Read the model definition and answer for the solid it produces. Units are mm, in the model's axes. Coordinates: 2 decimals unless noted, no trailing zeros. Write each loop counter-clockwise with the first axis right and the second up, starting at its lowest first coordinate (ties: lowest second). Pieces come first, ordered by that corner, then holes.
Item 1: Determine the mould class of faces 1 (the face through (1.02, 46.49, 1.97)), 2 (the face through (29.23, -26.81, 1.97)), 3 (the face through (-11, -10, 0)) for opening direction Y: released by +Y, released by -Y, zero draft, split by the parting line, or undercut.
Item 2: Each of these flat-tipped pins is pushed along its axis until it touches: P1, Ø3, axis at x = 28.28, y = 28.28, coming from the +Z side; P2, Ø1, axis at y = 22, z = 3, coming from the -X side; P3, Ø2, axis at y = 18.5, z = 3, coming from the +X side. Where does it stop, or does it pass through?
Item 3: Section C-C (y = 24) is taken. Give the vertices of the cut face in (x, z).
Item 4: Section A-A (x = -20) is taken. Give the vertices of the cut face in (y, z), then the cut area to 3 significant figures.
Item 5: Straight lines are drawn through the part: probe 1 along X at (y, z) = (-28, 3.55); probe 2 along Y at (x, z) = (-28.5, 0.35); probe 3 along X at (y, z) = (-40.5, 0.65). For each, find the intervals that lie inside material, in ascending order.
Item 6: Section B-B (z = 0.7) is taken. State how many separate pieces and enclosed holes the cut face has, then the cut area to 3 significant figures.
Item 7: Section D-D (y = 14) is taken. Give the vertices of the cut face in (x, z), then the cut area to 3 significant figures.
from build123d import *

# Parameters (mm, degrees)
SKETCH1_R           = 2.1
SKETCH1_R_2         = 12.5
SKETCH1_R_3         = 1.75
BOSS_EXTRUDE1_DEPTH = 4


with BuildPart() as part:
    # Sketch1 → Boss-Extrude1 (new body)
    with BuildSketch(Plane.XY):
        with BuildLine():
            Line((-46.5, 0), (-46.5, -46.5))
            Line((-46.5, -46.5), (46.5, -46.5))
            Line((46.5, -46.5), (46.5, 0))
            ThreePointArc((46.5, 0), (0, 46.5), (-46.5, 0))
        make_face()
        with Locations((0, 24)):
            Circle(SKETCH1_R, mode=Mode.SUBTRACT)
        with Locations((-20.784609691, -12)):
            Circle(SKETCH1_R, mode=Mode.SUBTRACT)
        with Locations((20.784609691, -12)):
            Circle(SKETCH1_R, mode=Mode.SUBTRACT)
        Circle(SKETCH1_R_2, mode=Mode.SUBTRACT)
        with Locations((0, 40)):
            Circle(SKETCH1_R_3, mode=Mode.SUBTRACT)
        with Locations((28.284271247, 28.284271247)):
            Circle(SKETCH1_R_3, mode=Mode.SUBTRACT)
        with Locations((40, 0)):
            Circle(SKETCH1_R_3, mode=Mode.SUBTRACT)
        with Locations((28.284271247, -28.284271247)):
            Circle(SKETCH1_R_3, mode=Mode.SUBTRACT)
        with Locations((0, -40)):
            Circle(SKETCH1_R_3, mode=Mode.SUBTRACT)
        with Locations((-28.284271247, -28.284271247)):
            Circle(SKETCH1_R_3, mode=Mode.SUBTRACT)
        with Locations((-40, 0)):
            Circle(SKETCH1_R_3, mode=Mode.SUBTRACT)
        with Locations((-28.284271247, 28.284271247)):
            Circle(SKETCH1_R_3, mode=Mode.SUBTRACT)
    extrude(amount=BOSS_EXTRUDE1_DEPTH)


solid = part.part
Established:
1. face 1: released by +Y
1. face 2: undercut
1. face 3: zero draft
2. P1: passes through
2. P2: stops at x = -41.23
2. P3: stops at x = 43.08
3. outline: (-39.83, 0) - (-2.1, 0) - (-2.1, 4) - (-39.83, 4) - close; (2.1, 0) - (39.83, 0) - (39.83, 4) - (2.1, 4) - close
4. outline: (-46.5, 0) - (-13.95, 0) - (-13.95, 4) - (-46.5, 4) - close; (-10.05, 0) - (41.98, 0) - (41.98, 4) - (-10.05, 4) - close
4. area: 338 mm2
5. probe 1: x = -46.5 to -30.01, -26.56 to 26.56, 30.01 to 46.5
5. probe 2: y = -46.5 to -30.02, -26.55 to 26.55, 30.02 to 36.74
5. probe 3: x = -46.5 to -1.68, 1.68 to 46.5
6. separate pieces: 1
6. enclosed holes: 12
6. area: 7,110 mm2
7. outline: (-44.34, 0) - (44.34, 0) - (44.34, 4) - (-44.34, 4) - close
7. area: 355 mm2
